The model under review builds one solid part; all positions refer to its coordinate system, in mm. A direction names the side the tool comes from. Round coordinates to 2 decimals unless told otherwise and drop trailing zeros. Write each loop counter-clockwise with the first axis right and the second up, starting at its lowest first coordinate (ties: lowest second). Pieces come first, ordered by that corner, then holes.
Item 1: Add section A-A (y = 0). Give the boundary of the cut face in (x, z).
Item 2: Clearance check with flat-ended pins moving along their axes: pin 1 Ø0.6 at (y, z) = (-15, 0.5) entering from -X; pin 2 Ø0.6 at (x, z) = (41, 1) entering from -Y; pin 3 Ø1 at (x, z) = (38.5, 1.5) entering from +Y; pin 4 Ø5.5 at (x, y) = (6.76, 11.72) entering from -Z. State where each tip first meets the part, or that it passes through.
Item 3: Add section B-B (x = 0). Give the boundary of the cut face in (y, z), plus the area to 3 significant figures.
Item 4: Add section C-C (y = 7.5). Give the boundary of the cut face in (x, z), plus the area to 3 significant figures.
Item 5: To check wall thickness, follow L1, parallel to Y at x = 0, z = 1; L2, parallel to Y at x = -33.5, z = 1.6; L3, parallel to X at y = 7, z = 1.9. State the ranges of each line that lie inside material, in increasing order.
Item 6: Machinability: for faces 4 (the face through (-30, 18, 1)), 5 (the face through (-39.5, 15, 1)), 6 (the face through (31.4, 0, 1)), 7 (the face through (33, -20, 1)), 8 (the face through (36, 3, 1)), which of the approach directions +Z, -Z, +X, -X, +Y, -Y give a long, thin tool a straight path to every point of the face, cutting with its end or side? Answer none if there is none.
Item 7: Add section D-D (z = 1.5). State how many separate pieces and enclosed holes the cut face has, plus the area to 3 significant figures.
Item 8: Draft analysis for pull direction X (two halves, no side actions). For faces 1 (the face through (30, -18, 1)), 2 (the face through (38, -17, 1)), 3 (the face through (-31.4, 0, 1)), state which applies: +X half, -X half, draft (parallel to the pull), parting line (faces both ways), or undercut.
```python
from build123d import *

# Parameters (mm, degrees)
SKETCH_1_R      = 2
SKETCH_1_R_2    = 2.08
SKETCH_1_R_3    = 8.75
EXTRUDE_2_DEPTH = 2


with BuildPart() as part:
    # 草图1 → 凸台-拉伸2 (new body)
    with BuildSketch(Plane.XY):
        with BuildLine():
            Line((-39.5, -13.75), (-39.5, -16))
            ThreePointArc((-39.5, -16), (-39.207106781, -16.707106781), (-38.5, -17))
            Line((-38.5, -17), (-37, -17))
            Line((-37, -17), (-37, -20))
            Line((-37, -20), (-30, -20))
            Line((-30, -20), (-30, -17))
            Line((-30, -17), (-25.488968202, -17))
            ThreePointArc((-25.488968202, -17), (0, -27.55787632), (25.488968202, -17))
            Line((25.488968202, -17), (30, -17))
            Line((30, -17), (30, -20))
            Line((30, -20), (37, -20))
            Line((37, -20), (37, -17))
            Line((37, -17), (39.5, -17))
            Line((39.5, -17), (39.5, -13.75))
            Line((39.5, -13.75), (42.5, -13.75))
            Line((42.5, -13.75), (42.5, -8.75))
            Line((42.5, -8.75), (39.5, -8.75))
            Line((39.5, -8.75), (39.5, -1.5))
            Line((39.5, -1.5), (37, -1.5))
            Line((37, -1.5), (37, -3))
            Line((37, -3), (34.4, -3))
            Line((34.4, -3), (34.4, -1.5))
            Line((34.4, -1.5), (31.4, -1.5))
            Line((31.4, -1.5), (31.4, 1.5))
            Line((31.4, 1.5), (34.4, 1.5))
            Line((34.4, 1.5), (34.4, 3))
            Line((34.4, 3), (37, 3))
            Line((37, 3), (37, 1.5))
            Line((37, 1.5), (39.5, 1.5))
            Line((39.5, 1.5), (39.5, 8.75))
            Line((39.5, 8.75), (42.5, 8.75))
            Line((42.5, 8.75), (42.5, 13.75))
            Line((42.5, 13.75), (39.5, 13.75))
            Line((39.5, 13.75), (39.5, 17))
            Line((39.5, 17), (37, 17))
            Line((37, 17), (37, 20))
            Line((37, 20), (30, 20))
            Line((30, 20), (30, 17))
            Line((30, 17), (25.488968202, 17))
            ThreePointArc((25.488968202, 17), (0, 27.55787632), (-25.488968202, 17))
            Line((-25.488968202, 17), (-30, 17))
            Line((-30, 17), (-30, 20))
            Line((-30, 20), (-37, 20))
            Line((-37, 20), (-37, 17))
            Line((-37, 17), (-39.5, 17))
            Line((-39.5, 17), (-39.5, 13.75))
            Line((-39.5, 13.75), (-42.5, 13.75))
            Line((-42.5, 13.75), (-42.5, 8.75))
            Line((-42.5, 8.75), (-39.5, 8.75))
            Line((-39.5, 8.75), (-39.5, 1.5))
            Line((-39.5, 1.5), (-37, 1.5))
            Line((-37, 1.5), (-37, 3))
            Line((-37, 3), (-34.4, 3))
            Line((-34.4, 3), (-34.4, 1.5))
            Line((-34.4, 1.5), (-31.4, 1.5))
            Line((-31.4, 1.5), (-31.4, -1.5))
            Line((-31.4, -1.5), (-34.4, -1.5))
            Line((-34.4, -1.5), (-34.4, -3))
            Line((-34.4, -3), (-37, -3))
            Line((-37, -3), (-37, -1.5))
            Line((-37, -1.5), (-39.5, -1.5))
            Line((-39.5, -1.5), (-39.5, -8.75))
            Line((-39.5, -8.75), (-42.5, -8.75))
            Line((-42.5, -8.75), (-42.5, -13.75))
            Line((-42.5, -13.75), (-39.5, -13.75))
        make_face()
        with Locations((0, -15)):
            Circle(SKETCH_1_R, mode=Mode.SUBTRACT)
        with Locations((-12.990381057, -7.5)):
            Circle(SKETCH_1_R, mode=Mode.SUBTRACT)
        with Locations((-12.990381057, 7.5)):
            Circle(SKETCH_1_R, mode=Mode.SUBTRACT)
        with Locations((0, 15)):
            Circle(SKETCH_1_R, mode=Mode.SUBTRACT)
        with Locations((12.990381057, 7.5)):
            Circle(SKETCH_1_R, mode=Mode.SUBTRACT)
        with Locations((12.990381057, -7.5)):
            Circle(SKETCH_1_R, mode=Mode.SUBTRACT)
        with Locations((-13.53, 0)):
            Circle(SKETCH_1_R_2, mode=Mode.SUBTRACT)
        with Locations((6.765, 11.717323713)):
            Circle(SKETCH_1_R_2, mode=Mode.SUBTRACT)
        with Locations((6.765, -11.717323713)):
            Circle(SKETCH_1_R_2, mode=Mode.SUBTRACT)
        Circle(SKETCH_1_R_3, mode=Mode.SUBTRACT)
    extrude(amount=EXTRUDE_2_DEPTH)


solid = part.part
```
Numbers:
1. outline: (-31.4, 0) - (-15.61, 0) - (-15.61, 2) - (-31.4, 2) - close; (-11.45, 0) - (-8.75, 0) - (-8.75, 2) - (-11.45, 2) - close; (8.75, 0) - (31.4, 0) - (31.4, 2) - (8.75, 2) - close
2. pin 1: stops at x = -39.5
2. pin 2: stops at y = -13.75
2. pin 3: stops at y = 17
2. pin 4: stops at z = 0
3. outline: (-27.56, 0) - (-17, 0) - (-17, 2) - (-27.56, 2) - close; (-13, 0) - (-8.75, 0) - (-8.75, 2) - (-13, 2) - close; (8.75, 0) - (13, 0) - (13, 2) - (8.75, 2) - close; (17, 0) - (27.56, 0) - (27.56, 2) - (17, 2) - close
3. area: 59.2 mm2
4. outline: (-39.5, 0) - (-14.99, 0) - (-14.99, 2) - (-39.5, 2) - close; (-10.99, 0) - (-4.51, 0) - (-4.51, 2) - (-10.99, 2) - close; (4.51, 0) - (10.99, 0) - (10.99, 2) - (4.51, 2) - close; (14.99, 0) - (39.5, 0) - (39.5, 2) - (14.99, 2) - close
4. area: 124 mm2
5. L1: y = -27.56 to -17, -13 to -8.75, 8.75 to 13, 17 to 27.56
5. L2: y = -20 to -1.5, 1.5 to 20
5. L3: x = -39.5 to -14.93, -11.05 to -5.25, 5.25 to 11.05, 14.93 to 39.5
6. face 4: +Z, -Z, +Y
6. face 5: +Z, -Z, -X, +Y
6. face 6: +Z, -Z, +X
6. face 7: +Z, -Z, +X, -Y
6. face 8: +Z, -Z
7. separate pieces: 1
7. enclosed holes: 10
7. area: 3,150 mm2
8. face 1: undercut
8. face 2: draft
8. face 3: -X half
